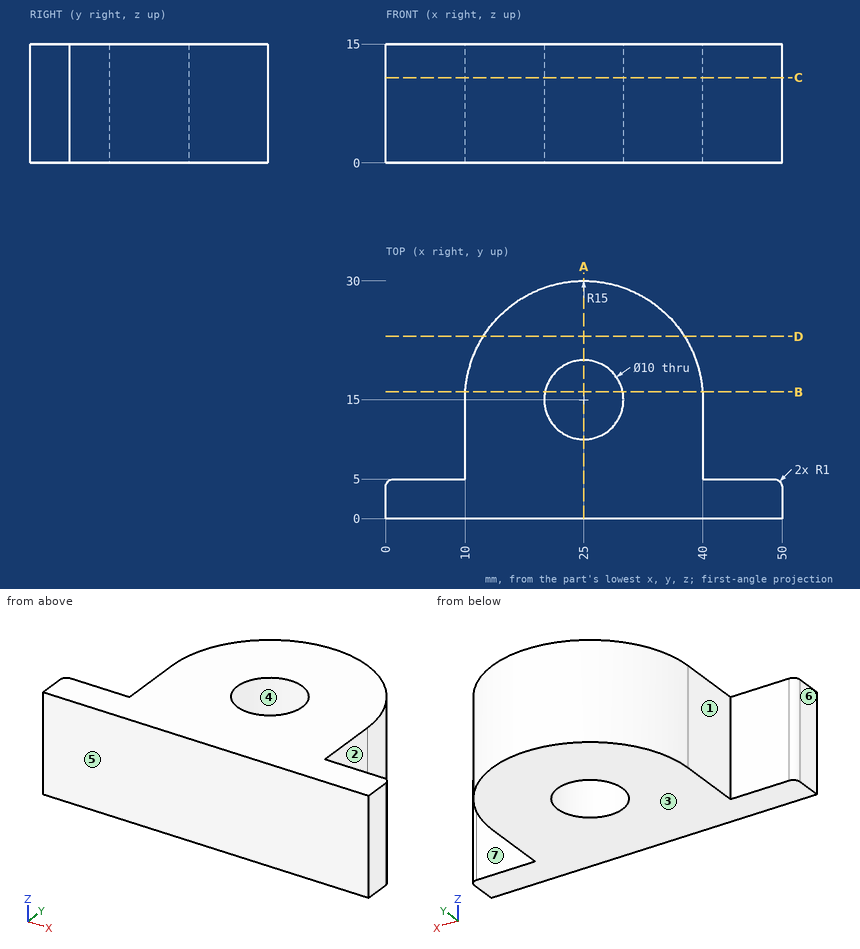
Could you check a few things on this drawing? It's one solid part, dimensions in mm from its lowest x, y, z. A direction names the side the tool comes from. Round coordinates to 2 decimals unless told otherwise and drop trailing zeros. Order: outer loops, then holes, each group sorted by start corner. A loop starts at its lowest first (then second) coordinate and runs counter-clockwise, first axis right, second up. Notation, with made-up numbers: M -16.5,66 L -0.5,66 A8 cw -0.5,75 Z; hole C 46.5,5.25 d7. An arc over 180 degrees is marked long. One line per question, with ' | ' between items.
1) I need wall thicknesses on line 1 (Y direction, x = 25, z = 8); line 2 (X direction, y = 14.75, z = 3.75); line 3 (X direction, y = 11, z = 14.25). Which ranges of each line are inside material? Lowest first, please.
Checked values:
line 1: y = 0 to 10, 20 to 30 | line 2: x = 10 to 20.01, 29.99 to 40 | line 3: x = 10 to 22, 28 to 40
2) We'd pull the mould along Y, two halves only. Please class the marked faces 4, 5, 6 and 7: released by +Y, released by -Y, zero draft, split by the parting line, or undercut.
Checked values:
face 4: undercut | face 5: released by -Y | face 6: zero draft | face 7: released by +Y
3) Imagine slicing it at C-C, the plane z = 10.75. Write out the boundary of the cut face in (x, y), plus the area to 3 significant figures.
Checked values:
outline: M 0,0 L 50,0 L 50,4 A1 ccw 49,5 L 40,5 L 40,15 A15 ccw 10,15 L 10,5 L 1,5 A1 ccw 0,4 Z; hole C 25,15 d10 | area: 824 mm²
4) Imagine slicing it at D-D, the plane y = 23. Write out the boundary of the cut face in (x, z), plus the area to 3 significant figures.
Checked values:
outline: M 12.31,0 L 37.69,0 L 37.69,15 L 12.31,15 Z | area: 381 mm²
5) Imagine slicing it at A-A, the plane x = 25. Write out the boundary of the cut face in (y, z).
Checked values:
outline: M 0,0 L 10,0 L 10,15 L 0,15 Z; M 20,0 L 30,0 L 30,15 L 20,15 Z
6) On a 3-axis mill with a long thin cutter (end or side, diameter ignored), from which of +Z, -Z, +X, -X, +Y, -Y can I reach the whole of each face in a straight line? I mean the marked faces 1, 2 and 3. Say none if no direction works.
Checked values:
face 1: +Z, -Z, -X, +Y | face 2: +Z, -Z, +X, +Y | face 3: -Z, +X, -X, +Y, -Y
7) Imagine slicing it at B-B, the plane y = 16. Write out the boundary of the cut face in (x, z), plus the area to 3 significant figures.
Checked values:
outline: M 10.03,0 L 20.1,0 L 20.1,15 L 10.03,15 Z; M 29.9,0 L 39.97,0 L 39.97,15 L 29.9,15 Z | area: 302 mm²
8) I'm going to push flat-ended pins straight in: pin 1 Ø8 at (x, z) = (42, 12.5) entering from +Y; pin 2 Ø8 at (y, z) = (10, 7) entering from -X; pin 3 Ø1 at (x, z) = (44.5, 10) entering from +Y. Where does each tip first touch, or does it pass through?
Checked values:
pin 1: stops at y = 22.48 | pin 2: stops at x = 10 | pin 3: stops at y = 5
